Design review of the part built by this model. Coordinates are the model's own, in mm. Coordinates: 2 decimals unless noted, no trailing zeros. Write each loop counter-clockwise with the first axis right and the second up, starting at its lowest first coordinate (ties: lowest second). Pieces come first, ordered by that corner, then holes. Notation, with made-up numbers: (32.25, 15.25) -> (77.25, 15.25) arc R36 ccw to (77.25, 49.25) -> close; hole circle Ø4 at (4.5, 6). An arc over 180 degrees is marked (long way). One line per question, with ' | ' between items. Start each with the question number.
Q1. Wall thickness on probe 1 along Z at (x, y) = (-43.5, 63.5); probe 2 along Y at (x, z) = (-30.5, -29.5); probe 3 along X at (y, z) = (56, -195.5): over which ranges is each line inside the solid? List them lowest first.
Q2. For P1, Ø20.5, axis at x = -31.5, y = 70, coming from the -Z side; P2, Ø6, axis at x = -32.5, y = 64, coming from the +Z side, all flat-tipped, find the tip position at first contact; note any pin that passes through.
Q3. Add section A-A on x = -42. State the section outline as (y, z) points.
Q4. Add section D-D on x = -18.5. State the section outline as (y, z) points.
Q5. Add section C-C on y = 55.5. State the section outline as (x, z) points, and give its area (3 significant figures).
Q6. Add section B-B on z = -212. State the section outline as (x, y) points, and give its area (3 significant figures).
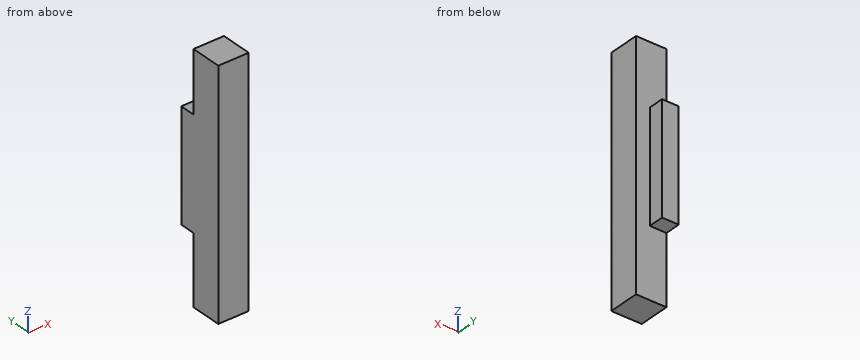
Autodesk Inventor part; units mm, degrees
ref_plane "YZ Plane" through (0, 0, 0) normal (1, 0, 0) x (0, 1, 0)
ref_plane "XZ Plane" through (0, 0, 0) normal (0, 1, 0) x (-1, 0, 0)
ref_plane "XY Plane" through (0, 0, 0) normal (0, 0, 1) x (1, 0, 0)
sketch "Sketch1" plane through (0, 0, 0) normal (0, 1, 0) x (-1, 0, 0)
  line L0 (0, 0) -> (50.8, 0)
  line L1 (50.8, 0) -> (50.8, -400)
  line L2 (50.8, -400) -> (0, -400)
  line L3 (0, -400) -> (0, 0)
  dimension "d0" = 50.8
  dimension "d1" = 400
extrude "Extrusion1" add sketch "Sketch1" along normal blind 77.8
sketch "Sketch3" plane through (0, 0, 0) normal (1, 0, 0) x (0, 0, -1)
  line L0 (0, 77.8) -> (101.6, 77.8)
  line L1 (101.6, 77.8) -> (101.6, 52)
  line L2 (101.6, 52) -> (0, 52)
  line L3 (0, 52) -> (0, 77.8)
  line L4 (0, 77.8) -> (400, 77.8)
  line L5 (400, 77.8) -> (285, 77.8)
  line L6 (285, 77.8) -> (285, 52)
  line L7 (285, 52) -> (400, 52)
  line L8 (400, 52) -> (400, 77.8)
  point P0 (0, 0)
  dimension "d8" = 101.6
  dimension "d9" = 25.8
  dimension "d10" = 115
  dimension "d11" = 25.8
extrude "Extrusion2" cut sketch "Sketch3" against normal blind 50.8
sketch "Sketch4" plane through (0, 77.8, 0) normal (0, 1, 0) x (1, 0, 0)
  line L0 (0, 101.6) -> (0, 285)
  line L1 (0, 285) -> (-50.8, 285)
  line L2 (0, 101.6) -> (-23, 101.6)
  line L3 (-23, 101.6) -> (-23, 285)
  line L4 (-23, 285) -> (0, 285)
  line L5 (0, 285) -> (0, 101.6)
  point P0 (0, 0)
  dimension "d14" = 23
extrude "Extrusion3" cut sketch "Sketch4" against normal blind 25.8
properties part number "PiezaPuerta-1"
Output values:
1) probe 1: z = -285 to -101.6 | probe 2: y = 0 to 52 | probe 3: x = -50.8 to -23
2) P1: stops at z = -285 | P2: stops at z = -101.6
3) outline: (0, -400) -> (52, -400) -> (52, -285) -> (77.8, -285) -> (77.8, -101.6) -> (52, -101.6) -> (52, 0) -> (0, 0) -> close
4) outline: (0, -400) -> (52, -400) -> (52, 0) -> (0, 0) -> close
5) outline: (-50.8, -285) -> (-23, -285) -> (-23, -101.6) -> (-50.8, -101.6) -> close | area: 5,100 mm2
6) outline: (-50.8, 0) -> (0, 0) -> (0, 52) -> (-23, 52) -> (-23, 77.8) -> (-50.8, 77.8) -> close | area: 3,360 mm2
